CAD build for the part. Positions are in the model's coordinates, mm. A direction names the side the tool comes from. Round coordinates to 2 decimals unless told otherwise and drop trailing zeros. Write each loop counter-clockwise with the first axis right and the second up, starting at its lowest first coordinate (ties: lowest second). Pieces come first, ordered by that corner, then holes. Notation, with made-up numbers: (42.25, 82.25) - (64.25, 82.25) arc R18 ccw to (64.25, 112.25) - close; hole circle Ø2 at (-31.5, 69.25). An arc over 180 degrees is marked (long way). Answer in a Markdown table with one row per item.
Autodesk Inventor part; units mm, degrees
ref_plane "to_left_XY" through (0, 0, 4.8387) normal (0, 1, 0) x (1, 0, 0)
ref_plane "to_left_YZ" through (0, 0, 4.8387) normal (1, 0, 0) x (0, 0, -1)
ref_plane "to_left_ZX" through (0, 0, 4.8387) normal (0, 0, -1) x (0, 1, 0)
sketch "Sketch_1" plane through (0, 0, 0) normal (0, 1, 0) x (-1, 0, 0)
  arc A0 (0, 0) -> (-4.8387, 4.8387) centre (0, 4.8387) ccw
  line L0 (-4.8387, 4.8387) -> (-4.8387, 2.5527)
  line L1 (-4.8387, 2.5527) -> (-2.4765, 2.5527)
  line L2 (-2.4765, 2.5527) -> (-2.4765, 4.8387)
  arc A1 (0, 2.3622) -> (-2.4765, 4.8387) centre (0, 4.8387) ccw
  line L3 (0, 2.3622) -> (-25.4, 2.3622)
  line L4 (-25.4, 2.3622) -> (-25.4, 0)
  line L5 (-25.4, 0) -> (0, 0)
extrude "Extrusion1" add sketch "Sketch_1" along normal mid plane 50.8
sketch "Sketch_2" plane through (0, 0, 0) normal (0, 0, 1) x (1, 0, 0)
  line L0 (-25.4, 50.8) -> (-25.4, -50.8)
  line L1 (-25.4, -50.8) -> (50.8, -50.8)
  line L2 (50.8, -50.8) -> (50.8, 50.8)
  line L3 (50.8, 50.8) -> (-25.4, 50.8)
  line L4 (-12.7, -0.0254) -> (-12.7, -25.4)
  line L5 (-12.7, -25.4) -> (19.05, -25.4)
  arc A0 (19.05, -25.4) -> (25.4, -19.05) centre (19.05, -19.05) ccw
  line L6 (25.4, -19.05) -> (25.4, 19.05)
  arc A1 (25.4, 19.05) -> (19.05, 25.4) centre (19.05, 19.05) ccw
  line L7 (19.05, 25.4) -> (5.0673, 25.4)
  line L8 (5.0673, 25.4) -> (5.0673, -0.0254)
  line L9 (5.0673, -0.0254) -> (-12.7, -0.0254)
extrude "Extrusion2" cut sketch "Sketch_2" along normal mid plane 25.4
sketch "Sketch_4" plane through (0, 0, 0) normal (0, 0, 1) x (1, 0, 0)
  circle A0 centre (13.4874, 12.7) radius 3.5687
extrude "Extrusion3" cut sketch "Sketch_4" along normal mid plane 4.7244
sketch "Sketch_5" plane through (0, 0, 0) normal (0, 0, 1) x (1, 0, 0)
  circle A0 centre (13.4874, -12.7) radius 3.5687
extrude "Extrusion4" cut sketch "Sketch_5" along normal mid plane 4.7244
ref_plane "to_left_XY" through (0, 0, 4.8387) normal (0, 1, 0) x (1, 0, 0)
ref_plane "to_left_YZ" through (0, 0, 4.8387) normal (1, 0, 0) x (0, 0, -1)
ref_plane "to_left_ZX" through (0, 0, 4.8387) normal (0, 0, -1) x (0, 1, 0)
properties part number "2838_right"
Q1. Saw through at B-B on z = 4.25. List the corners of the cut face in (x, y).
Computed:
| item | result |
|---|---|
| outline | (-4.8, -25.4) - (-2.41, -25.4) - (-2.41, -0.03) - (-4.8, -0.03) - close; (2.48, -25.4) - (4.84, -25.4) - (4.84, -0.03) - (2.48, -0.03) - close |
Q2. Drill centre lines: line 1 (Z direction, x = 20.5, y = 12.5); line 2 (Y direction, x = 3.5, z = 5.5); line 3 (X direction, y = -19.5, z = 5). Where is each one in solid material? Low to high.
Computed:
| item | result |
|---|---|
| line 1 | z = 0 to 2.36 |
| line 2 | y = -25.4 to -0.03 |
| line 3 | x = -4.84 to -2.47, 2.47 to 4.84 |
Q3. Pull direction Z, two halves, no side cores. Call faces 5 (the flat face through (4, -13, 2.553)), 6 (the flat face through (13, 0, 0)), 7 (the cylindrical face through (16.89, 11.63, 1.16)), 8 (the cylindrical face through (-3.31, -12.89, 8.37)): released by +Z, released by -Z, zero draft, split by the parting line, or undercut.
Computed:
| item | result |
|---|---|
| face 5 | undercut |
| face 6 | released by -Z |
| face 7 | zero draft |
| face 8 | split by the parting line |
Q4. 3-axis set-ups, long thin cutter, end or side, ignore diameter. For faces 1 (the flat face through (4.839, -13, 4)), 2 (the flat face through (2.476, -13, 4)), 3 (the flat face through (5.067, 13, 1)), 4 (the flat face through (13, 0, 2.362)): which of +Z, -Z, +X, -X, +Y, -Y reach the whole face in a straight line?
Computed:
| item | result |
|---|---|
| face 1 | +Z, +X, +Y, -Y |
| face 2 | +Y, -Y |
| face 3 | +Z, -Z, -X, +Y |
| face 4 | +X, +Y, -Y |
Q5. Flat gauge pins, fed straight in: pin 1 (11.5 mm diameter, centred on x = 13.49, y = -12.7, fed in from +Z); pin 2 (3 mm diameter, centred on y = 8.5, z = 4.5, fed in from -X); pin 3 (1.1 mm diameter, centred on y = -9, z = 4, fed in from -X); pin 4 (1.8 mm diameter, centred on y = -18.5, z = 4, fed in from +X). Where does each tip first touch, or does it go through?
Computed:
| item | result |
|---|---|
| pin 1 | stops at z = 2.36 |
| pin 2 | passes through |
| pin 3 | stops at x = -4.83 |
| pin 4 | stops at x = 4.84 |
Q6. Saw through at A-A on y = -12.7. List the corners of the cut face in (x, z).
Computed:
| item | result |
|---|---|
| outline | (0, 0) - (9.92, 0) - (9.92, 2.36) - (0, 2.36) arc R2.48 cw (long way) to (2.48, 4.84) - (2.48, 2.55) - (4.84, 2.55) - (4.84, 4.84) arc R4.84 ccw (long way) to start; (17.06, 0) - (25.4, 0) - (25.4, 2.36) - (17.06, 2.36) - close |
Q7. Saw through at D-D on y = -6.5. List the corners of the cut face in (x, z), then the cut area to 3 significant figures.
Computed:
| item | result |
|---|---|
| outline | (0, 0) - (25.4, 0) - (25.4, 2.36) - (0, 2.36) arc R2.48 cw (long way) to (2.48, 4.84) - (2.48, 2.55) - (4.84, 2.55) - (4.84, 4.84) arc R4.84 ccw (long way) to start |
| area | 106 mm2 |
Q8. Saw through at C-C on x = 16. List the corners of the cut face in (y, z), then the cut area to 3 significant figures.
Computed:
| item | result |
|---|---|
| outline | (-25.4, 0) - (-15.23, 0) - (-15.23, 2.36) - (-25.4, 2.36) - close; (-10.17, 0) - (10.17, 0) - (10.17, 2.36) - (-10.17, 2.36) - close; (15.23, 0) - (25.4, 0) - (25.4, 2.36) - (15.23, 2.36) - close |
| area | 96.1 mm2 |
